Build history of the part. All positions in model axes, mm. A direction names the side the tool comes from. Give positions to 0.01 mm unless a question says otherwise; leave off trailing zeros. Loops run counter-clockwise (first coordinate to the right, second up) from the corner with the lowest first, then second, coordinate; pieces in that order, holes last. Notation, with made-up numbers: (19.5, -34) -> (45.5, -34) arc R33 cw to (45.5, 3) -> close; hole circle Ø4 at (-16.5, 89.5). An arc over 180 degrees is marked (long way). Answer as a JSON object with one key per item and string values. Group by question number.
Q1. Band-saw the part on B-B, the plane y = 89. Write the cut outline in (x, z), plus the area to 4 significant figures.
Q2. Band-saw the part on A-A, the plane z = -6. Write the cut outline in (x, y).
Q3. Tool access for faces 1 (the flat face through (43.41, 110.94, 12.53)), 2 (the flat face through (1.5, 86, 6)), 3 (the flat face through (54, 60, -27)), 4 (the flat face through (30, 3, 12)): list every direction of +Z, -Z, +X, -X, +Y, -Y with a clear straight run to the whole face (end or side of a thin tool).
Q4. Drop flat-ended pins along their axis: pin 1 (3.5 mm diameter, centred on x = 31.5, z = 6.5, fed in from -Y); pin 2 (1.5 mm diameter, centred on x = 41, y = 1.5, fed in from +Z); pin 3 (2.5 mm diameter, centred on x = 45, y = 114.5, fed in from +Z); pin 4 (0.8 mm diameter, centred on x = 45, z = -4, fed in from -Y). Give the stop position or say it passes through.
Q5. Two-plate mould, pull along X, no slides. Class faces 5 (the flat face through (30, 5, 6)), 6 (the flat face through (0, 59, 7)), 7 (the flat face through (30, 120, 7)): pulls with the +X half, pulls with the -X half, needs draft (parallel to the pull), parting line crosses it, or undercut.
Q6. Band-saw the part on D-D, the plane y = 114.5. Write the cut outline in (x, z).
Q7. Band-saw the part on C-C, the plane x = 32.5. Write the cut outline in (y, z).
Q8. Wall check: probe 1 along Y at (x, z) = (21, 9.5); probe 2 along X at (y, z) = (114.5, 8); probe 3 along Y at (x, z) = (50.5, 10.5). Give the ranges that are in metal, low to high. Write a range as from..to.
Autodesk Inventor part; units mm, degrees
ref_plane "YZ Plane" through (0, 0, 0) normal (1, 0, 0) x (0, 1, 0)
ref_plane "XZ Plane" through (0, 0, 0) normal (0, 1, 0) x (-1, 0, 0)
ref_plane "XY Plane" through (0, 0, 0) normal (0, 0, 1) x (1, 0, 0)
sketch "Sketch1" plane through (0, 0, 0) normal (0, 0, 1) x (1, 0, 0)
  line L0 (0, 0) -> (0, 120)
  line L1 (0, 120) -> (61, 120)
  line L2 (61, 120) -> (61, 0)
  line L3 (61, 0) -> (0, 0)
  line L4 (0, 5) -> (61, 5)
  line L5 (0, 110) -> (61, 110)
  dimension "d0" = 120
  dimension "d1" = 61
  dimension "d14" = 10
  dimension "d15" = 5
extrude "Extrusion1" add sketch "Sketch1" along normal blind 14.5 contours L0 L5 L2 L4 | L0 L1 L2 L5
extrude "Extrusion2" cut sketch "Sketch1" along normal blind 11.5 contours L0 L5 L2 L4
extrude "Extrusion3" add sketch "Sketch1" along normal blind 12 contours L0 L4 L2 L3
sketch "Sketch2" plane through (61, 5, 14.5) normal (1, 0, 0) x (0, 0, -1)
  line L0 (14.5, 115) -> (0, 115)
  line L1 (14.5, 115) -> (0, 115)
  line L2 (0, 0) -> (0, 115)
  line L3 (0, 115) -> (0, 0)
  line L4 (0, 0) -> (14.5, 0)
  line L5 (14.5, 0) -> (14.5, 115)
  point P0 (14.5, -5)
extrude "Extrusion4" add sketch "Sketch2" against normal blind 1.5
sketch "Sketch3" plane through (0, 5, 14.5) normal (-1, 0, 0) x (0, 0, 1)
  line L0 (-14.5, 115) -> (-14.5, 105)
  line L1 (-14.5, 115) -> (0, 115)
  line L2 (-14.5, 115) -> (0, 115)
  line L3 (0, 0) -> (0, 115)
  line L4 (0, 115) -> (0, 0)
  line L5 (0, 0) -> (-14.5, 0)
  line L6 (-14.5, 0) -> (-14.5, 115)
  point P0 (-14.5, -5)
extrude "Extrusion5" add sketch "Sketch3" against normal blind 1.5
sketch "Sketch4" plane through (0, 0, 14.5) normal (0, 0, 1) x (1, 0, 0)
  circle A0 centre (45, 114.5) radius 2.25
  line L0 (61, 120) -> (0, 120)
  line L1 (45, 116.75) -> (46.9486, 115.625)
  line L2 (46.9486, 115.625) -> (46.9486, 113.375)
  line L3 (46.9486, 113.375) -> (45, 112.25)
  line L4 (45, 112.25) -> (43.0514, 113.375)
  line L5 (43.0514, 113.375) -> (43.0514, 115.625)
  line L6 (43.0514, 115.625) -> (45, 116.75)
  line L7 (0, 120) -> (0, 5)
  point P0 (0, 0)
  point P1 (30.5, 120)
  dimension "d23" = 4.5
  dimension "d60" = 45
hole "Hole1" at (45, 114.5, 14.5) direction (0, 0, -1) diameter 4.5 end through all counterbore diameter 9 counterbore depth 4
sketch "Sketch8" plane through (0, 0, 11.5) normal (0, 0, -1) x (-1, 0, 0)
  line L0 (-59.5, 110) -> (-1.5, 110)
  line L1 (-45, 110) -> (-45, 93)
  circle A0 centre (-45, 93) radius 1.4
  line L2 (-46.4, 93) -> (-43.6, 93)
  circle A1 centre (-36, 60) radius 1.4
  circle A2 centre (-54, 60) radius 1.4
  line L3 (-61, 0) -> (-61, 120)
  line L4 (-59.5, 110) -> (-59.5, 5)
  point P0 (0, 0)
  dimension "d45" = 17
  dimension "d46" = 2.8
  dimension "d56" = 2.8
  dimension "d57" = 2.8
  dimension "d66" = 33
  dimension "d67" = 33
  dimension "d68" = 9
  dimension "d69" = 18
extrude "Extrusion8" add sketch "Sketch8" along normal blind 38.5 contours A0 L2 L1 | L1 L2 A0
sketch "Sketch9" plane through (0, 0, 14.5) normal (0, 0, 1) x (1, 0, 0)
  circle A0 centre (45, 114.5) radius 2.25
  circle A1 centre (45, 114.5) radius 4.5
  line L0 (48.665, 117.1111) -> (49.0938, 112.6316)
  line L1 (49.0938, 112.6316) -> (45.4288, 110.0205)
  line L2 (45.4288, 110.0205) -> (41.335, 111.8889)
  line L3 (41.335, 111.8889) -> (40.9062, 116.3684)
  line L4 (40.9062, 116.3684) -> (44.5712, 118.9795)
  line L5 (44.5712, 118.9795) -> (48.665, 117.1111)
  point P0 (0, 0)
  point P1 (45, 110)
  point P2 (44.5712, 118.9795)
  point P3 (44.5712, 118.9795)
  point P4 (40.9062, 116.3684)
  point P5 (40.9062, 116.3684)
  point P6 (41.335, 111.8889)
  point P7 (41.335, 111.8889)
  point P8 (49.0938, 112.6316)
  point P9 (45.4288, 110.0205)
  point P10 (49.0938, 112.6316)
  point P11 (45.4288, 110.0205)
  dimension "d53" = 8
extrude "Extrusion9" add sketch "Sketch9" against normal blind 4 contours A1 L0 | L5 A1 | L4 A1 | A1 L2 | L3 A1
extrude "Extrusion10" add sketch "Sketch9" against normal blind 4 contours A1 L1
sketch "Sketch10" plane through (45, 93, -27) normal (0, 0, -1) x (1, 0, 0)
  arc A0 (-1.4, 0) -> (1.4, 0) centre (0, 0) ccw
  line L0 (-1.4, 0) -> (1.4, 0)
  point P0 (-45, 93)
extrude "Extrusion11" add sketch "Sketch8" along normal blind 38.5 contours A2
sketch "Sketch11" plane through (1.5, 5, 14.5) normal (1, 0, 0) x (0, 0, -1)
  line L0 (3, 105) -> (14.5, 105)
  line L1 (3, 105) -> (3, 56.18)
  line L2 (3, 0) -> (3, 105)
  line L3 (3, 56.18) -> (14.5, 56.18)
  line L4 (14.5, 115) -> (14.5, -5)
  line L5 (14.5, 56.18) -> (14.5, 54.18)
  line L6 (14.5, 54.18) -> (3, 54.18)
  line L7 (3, 54.18) -> (3, 56.18)
  point P0 (3, 54.18)
  dimension "d70" = 48.82
  dimension "d71" = 2
extrude "Extrusion12" add sketch "Sketch11" along normal blind 47 contours L3 L4 L6 L2
properties part number "Cover of DC Housing_3DPrint"
Worked answers:
{
 "1": {"outline": "(0, 0) -> (1.5, 0) -> (1.5, 11.5) -> (59.5, 11.5) -> (59.5, 0) -> (61, 0) -> (61, 14.5) -> (0, 14.5) -> close", "area": "217.5 mm2"},
 "2": {"outline": "(43.6, 93) -> (46.4, 93) arc R1.4 ccw to start; circle Ø2.8 at (54, 60)"},
 "3": {"face 1": "+Z", "face 2": "-Z", "face 3": "-Z, +X, -X, +Y, -Y", "face 4": "+Z, +X, -X, -Y"},
 "4": {"pin 1": "y = 0", "pin 2": "z = 12", "pin 3": "through", "pin 4": "y = 93"},
 "5": {"face 5": "undercut", "face 6": "pulls with the -X half", "face 7": "needs draft"},
 "6": {"outline": "(0, 0) -> (42.75, 0) -> (42.75, 10.5) -> (41.09, 10.5) -> (41.09, 14.5) -> (0, 14.5) -> close; (47.25, 0) -> (61, 0) -> (61, 14.5) -> (48.91, 14.5) -> (48.91, 10.5) -> (47.25, 10.5) -> close"},
 "7": {"outline": "(0, 0) -> (5, 0) -> (5, 11.5) -> (59.18, 11.5) -> (59.18, 0) -> (61.18, 0) -> (61.18, 11.5) -> (110, 11.5) -> (110, 0) -> (120, 0) -> (120, 14.5) -> (5, 14.5) -> (5, 12) -> (0, 12) -> close"},
 "8": {"probe 1": "0..5, 59.18..61.18, 110..120", "probe 2": "0..42.75, 47.25..61", "probe 3": "0..5, 110..120"}
}
